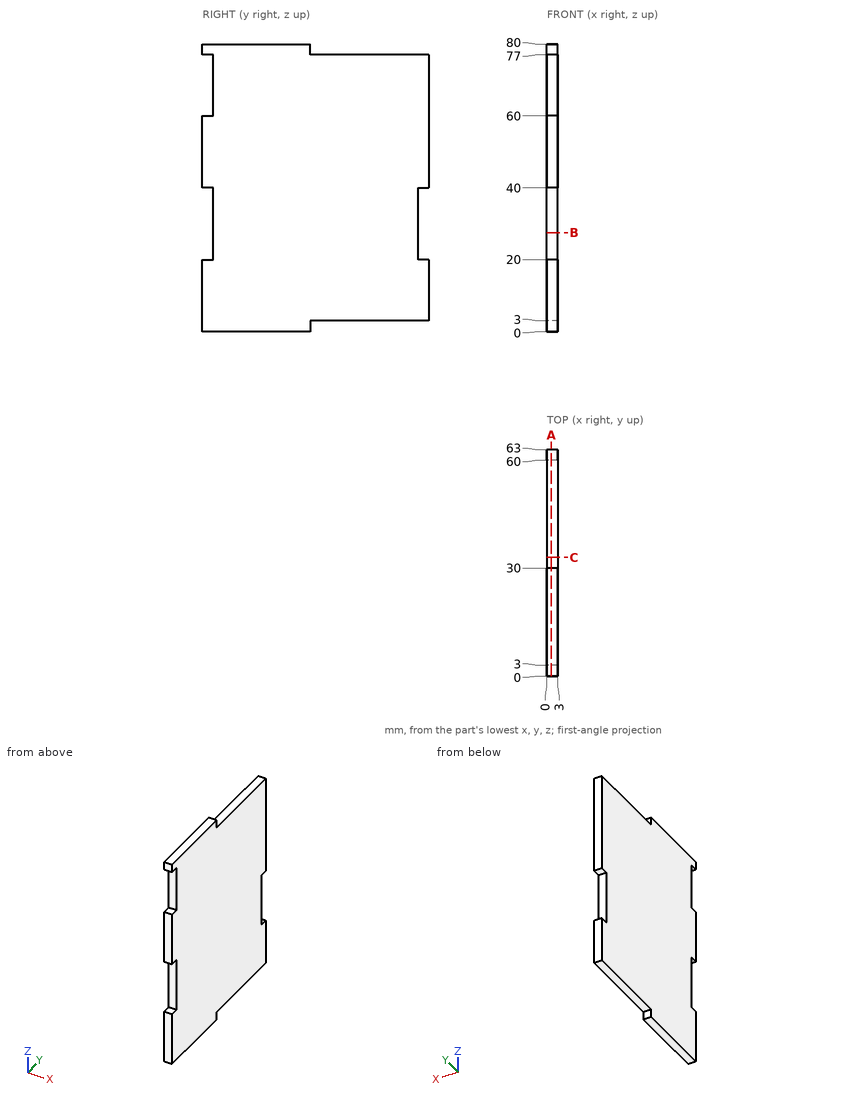
The figure shows three views and two pictorial views of one solid part (mm, origin at its lowest corner). Answer the questions. Give positions to 0.01 mm unless a question says otherwise; leave off trailing zeros. Order: outer loops, then holes, each group sorted by start corner. A loop starts at its lowest first (then second) coordinate and runs counter-clockwise, first axis right, second up. Notation, with made-up numbers: (22.5, 79) -> (63.5, 79) arc R32 ccw to (63.5, 114) -> close; hole circle Ø10 at (14.5, 3.5). An arc over 180 degrees is marked (long way). Answer as CSV lines item,"result". Start each with the question number.
Q1. Find the intervals of material crossed by L1, parallel to Y at x = 0.8, z = 39; L2, parallel to Z at x = 2.65, y = 51.5, in increasing order.
Q2. Given pin 1 (1.5 mm diameter, centred on x = 2, z = 69, fed in from -Y); pin 2 (1.5 mm diameter, centred on x = 1.5, y = 42.5, fed in from -Z); pin 3 (1.5 mm diameter, centred on x = 1, z = 35, fed in from +Y), each flat-ended and moving along its own axis, determine where each tip first touches the part or whether it passes through.
Q3. A cutting plane is placed at B-B (z = 27.5). Determine the outline of the cut face in (x, y).
Q4. A cutting plane is placed at C-C (y = 33). Determine the outline of the cut face in (x, z).
Q5. A cutting plane is placed at A-A (x = 1.25). Determine the outline of the cut face in (y, z).
Results found:
1,L1,"3 to 60"
1,L2,"3 to 77"
2,pin 1,"y = 3"
2,pin 2,"z = 3"
2,pin 3,"y = 60"
3,outline,"(0, 3) -> (3, 3) -> (3, 60) -> (0, 60) -> close"
4,outline,"(0, 3) -> (3, 3) -> (3, 77) -> (0, 77) -> close"
5,outline,"(0, 0) -> (30, 0) -> (30, 3) -> (63, 3) -> (63, 20) -> (60, 20) -> (60, 40) -> (63, 40) -> (63, 77) -> (30, 77) -> (30, 80) -> (0, 80) -> (0, 77) -> (3, 77) -> (3, 60) -> (0, 60) -> (0, 40) -> (3, 40) -> (3, 20) -> (0, 20) -> close"
